from build123d import *

# Parameters (mm, degrees)
SKETCH1_R           = 1.3335
SKETCH1_R_2         = 1.5875
BOSS_EXTRUDE1_DEPTH = 1.651
CHAMFER1_SIZE       = 2.54
SKETCH1_2_R         = 1.5875
BOSS_EXTRUDE2_DEPTH = 2.413
SKETCH1_3_R         = 1.5875
CUT_EXTRUDE1_DEPTH  = 0.889
SKETCH5_R           = 4.191
CUT_EXTRUDE5_DEPTH  = 23.382376376


with BuildPart() as part:
    # Sketch1 → Boss-Extrude1 (new body)
    with BuildSketch(Plane(origin=(0, 0, 0), x_dir=(1, 0, 0), z_dir=(0, 1, 0))):
        with BuildLine():
            Line((-5.567119422, 8.9535), (5.567119422, 8.9535))
            ThreePointArc((5.567119422, 8.9535), (6.35, 6.5405), (7.132880578, 8.9535))
            Line((7.132880578, 8.9535), (20.447, 8.9535))
            Line((20.447, 8.9535), (20.447, -8.9535))
            Line((20.447, -8.9535), (7.132880578, -8.9535))
            ThreePointArc((7.132880578, -8.9535), (6.35, -6.5405), (5.567119422, -8.9535))
            Line((5.567119422, -8.9535), (-5.567119422, -8.9535))
            ThreePointArc((-5.567119422, -8.9535), (-6.35, -6.5405), (-7.132880578, -8.9535))
            Line((-7.132880578, -8.9535), (-20.447, -8.9535))
            Line((-20.447, -8.9535), (-20.447, 8.9535))
            Line((-20.447, 8.9535), (-7.132880578, 8.9535))
            ThreePointArc((-7.132880578, 8.9535), (-6.35, 6.5405), (-5.567119422, 8.9535))
        make_face()
        with Locations(Location((-17.8308, 5.6769, 0), (0, 0, 90))):
            Circle(SKETCH1_R, mode=Mode.SUBTRACT)
        with Locations(Location((17.8308, 5.6769, 0), (0, 0, 90))):
            Circle(SKETCH1_R, mode=Mode.SUBTRACT)
        with Locations(Location((17.8308, -5.6769, 0), (0, 0, 90))):
            Circle(SKETCH1_R, mode=Mode.SUBTRACT)
        with Locations(Location((-17.8308, -5.6769, 0), (0, 0, 90))):
            Circle(SKETCH1_R, mode=Mode.SUBTRACT)
        with Locations(Location((-10.414, 5.6769, 0), (0, 0, 90))):
            Circle(SKETCH1_R_2, mode=Mode.SUBTRACT)
        with Locations(Location((10.414, 5.6769, 0), (0, 0, 90))):
            Circle(SKETCH1_R_2, mode=Mode.SUBTRACT)
        with Locations(Location((10.414, -5.6769, 0), (0, 0, 90))):
            Circle(SKETCH1_R_2, mode=Mode.SUBTRACT)
        with Locations(Location((-10.414, -5.6769, 0), (0, 0, 90))):
            Circle(SKETCH1_R_2, mode=Mode.SUBTRACT)
    extrude(amount=BOSS_EXTRUDE1_DEPTH)

    # Chamfer1
    chamfer1_edges = [part.edges().sort_by_distance(p)[0] for p in [
        (20.447, 0.8255, -8.9535),
        (20.447, 0.8255, 8.9535),
        (-20.447, 0.8255, 8.9535),
        (-20.447, 0.8255, -8.9535),
    ]]
    chamfer(chamfer1_edges, length=CHAMFER1_SIZE)

    # Sketch1_2 → Boss-Extrude2 (add)
    with BuildSketch(Plane(origin=(0, 0, 0), x_dir=(1, 0, 0), z_dir=(0, 1, 0))):
        with Locations(Location((-10.414, 5.6769, 0), (0, 0, 270))):
            Circle(SKETCH1_2_R)
        with Locations(Location((10.414, 5.6769, 0), (0, 0, 270))):
            Circle(SKETCH1_2_R)
        with Locations(Location((10.414, -5.6769, 0), (0, 0, 270))):
            Circle(SKETCH1_2_R)
        with Locations(Location((-10.414, -5.6769, 0), (0, 0, 270))):
            Circle(SKETCH1_2_R)
    extrude(amount=BOSS_EXTRUDE2_DEPTH)

    # Sketch1_3 → Cut-Extrude1 (cut)
    with BuildSketch(Plane(origin=(0, 0, 0), x_dir=(1, 0, 0), z_dir=(0, 1, 0))):
        with Locations(Location((-10.414, 5.6769, 0), (0, 0, 270))):
            Circle(SKETCH1_3_R)
        with Locations(Location((10.414, 5.6769, 0), (0, 0, 270))):
            Circle(SKETCH1_3_R)
        with Locations(Location((10.414, -5.6769, 0), (0, 0, 270))):
            Circle(SKETCH1_3_R)
        with Locations(Location((-10.414, -5.6769, 0), (0, 0, 270))):
            Circle(SKETCH1_3_R)
    extrude(amount=CUT_EXTRUDE1_DEPTH, mode=Mode.SUBTRACT)

    # Sketch5 → Cut-Extrude5 (cut, through all)
    with BuildSketch(Plane(origin=(0, 1.651, 0), x_dir=(1, 0, 0), z_dir=(0, 1, 0))):
        with Locations(Location((-14.0335, 0, 0), (0, 0, 270))):
            Circle(SKETCH5_R)
        with BuildLine():
            Line((6.106574162, -2.159), (11.705551547, -2.159))
            ThreePointArc((11.705551547, -2.159), (17.2085, 0), (11.705551547, 2.159))
            Line((11.705551547, 2.159), (6.106574162, 2.159))
            ThreePointArc((6.106574162, 2.159), (-6.477, 0), (6.106574162, -2.159))
        make_face()
    extrude(amount=-CUT_EXTRUDE5_DEPTH, mode=Mode.SUBTRACT)


solid = part.part
Could you check a few things on this model? Use its own coordinates, in mm. A direction names the side the tool comes from. Coordinates: 2 decimals unless noted, no trailing zeros. Order: outer loops, then holes, each group sorted by start corner. A loop starts at its lowest first (then second) coordinate and runs counter-clockwise, first axis right, second up. Notation, with made-up numbers: (-5.5, 63.25) - (13.5, 63.25) arc R24 ccw to (13.5, 100.25) - close; hole circle Ø8 at (58.5, 42.25). An arc over 180 degrees is marked (long way). Answer in a Markdown table with one row per item. Add a question column.
(1) I need wall thicknesses on L1, parallel to X at y = 0.45, z = 0; L2, parallel to Z at x = 10.5, y = 0.65; L3, parallel to Z at x = 0, y = 1.3. Which ranges of each line are inside material? Lowest first, please.
(2) If we section it at B-B, the plane z = 0: Please give me the cut outline in (x, y), then the cut area to 3 significant figures.
(3) If we mould it in two halves opening along Z, with no side actions, what happens to faces 4 (the face through (8.864, 2.027, -6.021)), 5 (the face through (-12, 1, 8.954)), 6 (the face through (-19.19, 0.81, -7.67)), 7 (the face through (10, 0.889, 6))? For each: released by +Z, released by -Z, zero draft, split by the parting line, or undercut.
(4) If we section it at C-C, the plane z = 5.5: State how many separate pieces and enclosed holes the cut face has, then the cut area to 3 significant figures.
(5) Will these pins go through, and if not, where does the flat tip stop? pin 1 (4.5 mm diameter, centred on x = -6.35, z = -7.874, fed in from +Y); pin 2 (8 mm diameter, centred on x = 4.5, z = 0, fed in from -Y); pin 3 (1 mm diameter, centred on x = -11, z = 6.5, fed in from -Y).
(6) On a 3-axis mill with a long thin cutter (end or side, diameter ignored), from which of +Z, -Z, +X, -X, +Y, -Y can I reach the whole of each face in a straight line? I mean faces 1 (the face through (9, 1, 2.159)), 2 (the face through (-9.94, 2.03, 7.19)), 3 (the face through (9.806, 0.438, 7.143)). Say none if no direction works.
(7) If we section it at A-A, the plane x = 0: Please give me the cut outline in (y, z).
(8) If we section it at D-D, the plane x = 11: Please give me the cut outline in (y, z).
Results are:
| question | item | result |
|---|---|---|
| 1 | L1 | x = -20.45 to -18.22, -9.84 to -6.48, 17.21 to 20.45 |
| 1 | L2 | z = -8.95 to -7.26, -4.09 to -2.16, 2.16 to 4.09, 7.26 to 8.95 |
| 1 | L3 | z = -8.95 to -6.48, 6.48 to 8.95 |
| 2 | outline | (-20.45, 0) - (-18.22, 0) - (-18.22, 1.65) - (-20.45, 1.65) - close; (-9.84, 0) - (-6.48, 0) - (-6.48, 1.65) - (-9.84, 1.65) - close; (17.21, 0) - (20.45, 0) - (20.45, 1.65) - (17.21, 1.65) - close |
| 2 | area | 14.6 mm2 |
| 3 | face 4 | undercut |
| 3 | face 5 | released by +Z |
| 3 | face 6 | released by -Z |
| 3 | face 7 | undercut |
| 4 | separate pieces | 4 |
| 4 | enclosed holes | 0 |
| 4 | area | 46.7 mm2 |
| 5 | pin 1 | stops at y = 1.65 |
| 5 | pin 2 | stops at y = 0 |
| 5 | pin 3 | stops at y = 0.89 |
| 6 | face 1 | +Y, -Y |
| 6 | face 2 | +Y |
| 6 | face 3 | -Y |
| 7 | outline | (0, -8.95) - (1.65, -8.95) - (1.65, -6.48) - (0, -6.48) - close; (0, 6.48) - (1.65, 6.48) - (1.65, 8.95) - (0, 8.95) - close |
| 8 | outline | (0, -8.95) - (1.65, -8.95) - (1.65, -7.15) - (2.41, -7.15) - (2.41, -4.2) - (1.65, -4.2) - (1.65, -2.16) - (0, -2.16) - (0, -4.2) - (0.89, -4.2) - (0.89, -7.15) - (0, -7.15) - close; (0, 2.16) - (1.65, 2.16) - (1.65, 4.2) - (2.41, 4.2) - (2.41, 7.15) - (1.65, 7.15) - (1.65, 8.95) - (0, 8.95) - (0, 7.15) - (0.89, 7.15) - (0.89, 4.2) - (0, 4.2) - close |
